Autodesk Inventor part; units mm, degrees
ref_plane "YZ Plane" through (0, 0, 0) normal (1, 0, 0) x (0, 1, 0)
ref_plane "XZ Plane" through (0, 0, 0) normal (0, 1, 0) x (-1, 0, 0)
ref_plane "XY Plane" through (0, 0, 0) normal (0, 0, 1) x (1, 0, 0)
sketch "Sketch1" plane through (0, 0, 0) normal (0, 1, 0) x (-1, 0, 0)
  line L0 (263.2333, -205.0309) -> (43.2333, -205.0309)
  line L1 (43.2333, -205.0309) -> (43.2333, -365.0309)
  line L2 (43.2333, -365.0309) -> (263.2333, -365.0309)
  line L3 (263.2333, -260.0309) -> (263.2333, -205.0309)
  line L4 (249.5333, -205.0309) -> (249.5333, -365.0309) construction
  line L5 (363.2333, -260.0309) -> (43.2333, -260.0309) construction
  line L6 (363.2333, -285.0309) -> (43.2333, -285.0309) construction
  line L7 (249.5333, -365.0309) -> (249.5333, -205.0309) construction
  line L8 (363.2333, -310.0309) -> (43.2333, -310.0309) construction
  line L9 (189.0333, -205.0309) -> (189.0333, -365.0309) construction
  circle A0 centre (249.5333, -260.0309) radius 2.55
  circle A1 centre (249.5333, -310.0309) radius 2.55
  circle A2 centre (189.0333, -260.0309) radius 2.55
  circle A3 centre (189.0333, -310.0309) radius 3.55
  line L10 (219.2833, -205.0309) -> (219.2833, -365.0309) construction
  circle A4 centre (219.2833, -285.0309) radius 1
  line L11 (263.2333, -205.0309) -> (363.2333, -205.0309)
  line L12 (363.2333, -205.0309) -> (363.2333, -365.0309)
  line L13 (363.2333, -365.0309) -> (263.2333, -365.0309)
  line L14 (363.2333, -230.0309) -> (43.2333, -230.0309) construction
  line L15 (363.2333, -340.0309) -> (43.2333, -340.0309) construction
  line L16 (363.2333, -214.7809) -> (270.7929, -214.7809) construction
  circle A5 centre (273.2333, -214.7809) radius 2.55
  line L17 (260.2333, -205.0309) -> (260.2333, -242.3907) construction
  circle A6 centre (273.2333, -245.2809) radius 2.55
  circle A7 centre (247.2333, -214.7809) radius 2.55
  circle A8 centre (247.2333, -245.2809) radius 2.55
  circle A9 centre (273.2333, -355.2809) radius 2.55
  circle A10 centre (273.2333, -324.7809) radius 2.55
  circle A11 centre (247.2333, -355.2809) radius 2.55
  circle A12 centre (247.2333, -324.7809) radius 2.55
  line L18 (163.2333, -205.0309) -> (163.2333, -365.0309) construction
  circle A13 centre (53.2333, -214.7809) radius 2.55
  circle A14 centre (53.2333, -245.2809) radius 2.55
  circle A15 centre (79.2333, -214.7809) radius 2.55
  circle A16 centre (79.2333, -245.2809) radius 2.55
  circle A17 centre (53.2333, -355.2809) radius 2.55
  circle A18 centre (53.2333, -324.7809) radius 2.55
  circle A19 centre (79.2333, -324.7809) radius 2.55
  circle A20 centre (79.2333, -355.2809) radius 2.55
  point P0 (0, 0)
  point P1 (263.2333, -310.0309)
  dimension "d2" = 13.7
  dimension "d4" = 60.5
  dimension "d5" = 5.1
  dimension "d6" = 5.1
  dimension "d7" = 5.1
  dimension "d8" = 7.1
  dimension "d11" = 2
  dimension "d15" = 50
  dimension "d17" = 100
  dimension "d18" = 25
  dimension "d19" = 15.25
  dimension "d20" = 5.1
  dimension "d21" = 13
  dimension "d22" = 90
  dimension "d23" = 160
  dimension "d24" = 110
  dimension "d27" = 320
extrude "Extrusion1" add sketch "Sketch1" along normal blind 3 contours L11 L12 L13 L2 L1 L0 | A4 | A5 | A6 | A7 | A8 | A9 | A10 | A11 | A12 | A13 | A14 | A15 | A16 | A17 | A18 | A19 | A20
sketch "Sketch2" plane through (0, 3, 0) normal (0, 1, 0) x (1, 0, 0)
  point P0 (0, 0)
extrude "Extrusion2" cut sketch "Sketch1" along normal through all contours A4
extrude "Extrusion3" cut sketch "Sketch1" along normal through all contours A5 | A6 | A7 | A8 | A9 | A10 | A11 | A12 | A13 | A14 | A15 | A16 | A17 | A18 | A19 | A20
properties part number "V Rail Gantry" material "Aluminum 6061"
Check sheet for the modelled part. Datum: model origin and axes. Units: mm. Coordinates: 2 decimals unless noted, no trailing zeros. Use one line per item in the form item = value.
Item 1: Material ranges on L1, parallel to Z at x = -275, y = 2.4; L2, parallel to Z at x = -188, y = 1.7; L3, parallel to Z at x = -218.5, y = 0.65, recorded low to high. Write a range as from..to.
Answer below:
L1 = -365.03..-357.12, -353.44..-326.62, -322.94..-247.12, -243.44..-216.62, -212.94..-205.03
L2 = -365.03..-313.43, -306.63..-262.36, -257.7..-205.03
L3 = -365.03..-285.65, -284.41..-205.03
Item 2: Release check for a two-part mould opening along Z. For faces 1 (the face through (-201, 3, -284)), 2 (the face through (-188.264, 1.479, -306.565)) record: pulls with the +Z half, pulls with the -Z half, needs draft (parallel to the pull), parting line crosses it, or undercut.
Answer below:
face_1 = needs draft
face_2 = undercut
Item 3: Gauge pin test, flat end, axial feed: pin 1 Ø4 at (x, z) = (-247.23, -214.78) entering from +Y. Record the tip position at first contact, or that the pin passes through.
Answer below:
pin_1 = through
